from build123d import *

# Parameters (mm, degrees)
BOSS_EXTRUDE1_DEPTH      = 15
BOSS_EXTRUDE1_DEPTH_BACK = 15
SKETCH4_R                = 1.5
BOSS_EXTRUDE2_DEPTH      = 15
BOSS_EXTRUDE2_DEPTH_BACK = 15
SKETCH6_R                = 1.5


with BuildPart() as part:
    # Sketch1 → Revolve1 (revolve)
    with BuildSketch(Plane.XY, mode=Mode.PRIVATE) as revolve1_sk:
        with BuildLine():
            Line((-7.75, 54.212646434), (-7.75, 30.212646434))
            Line((-7.75, 30.212646434), (-3, 12.850690899))
            Line((-3, 12.850690899), (0, 12.850690899))
            Line((0, 12.850690899), (0, 67.181279304))
            ThreePointArc((0, 67.181279304), (-7.553938352, 62.895480825), (-7.75, 54.212646434))
        make_face()
    revolve(revolve1_sk.sketch.rotate(Axis((0, 0, 0), (0, 1, 0)), 270), axis=Axis((0, 0, 0), (0, 1, 0)))

    # Sketch4 → Boss-Extrude1 (add, two sides: drawn at the far end of the back side and taken through both)
    with BuildSketch(Plane.XY.offset(-BOSS_EXTRUDE1_DEPTH_BACK)):
        with Locations((0, 58.381279304)):
            Circle(SKETCH4_R)
    extrude(amount=BOSS_EXTRUDE1_DEPTH + BOSS_EXTRUDE1_DEPTH_BACK)

    # Sketch6 → Boss-Extrude2 (add, two sides: drawn at the far end of the back side and taken through both)
    with BuildSketch(Plane(origin=(0, 0, 0), x_dir=(0, 0, -1), z_dir=(1, 0, 0)).offset(-BOSS_EXTRUDE2_DEPTH_BACK)):
        with Locations((0, 58.381279304)):
            Circle(SKETCH6_R)
        with Locations((3, 47.381279304)):
            Circle(SKETCH6_R)
        with Locations((-3, 47.381279304)):
            Circle(SKETCH6_R)
    extrude(amount=BOSS_EXTRUDE2_DEPTH + BOSS_EXTRUDE2_DEPTH_BACK)


solid = part.part
Input: part model. Units: mm. Frame: model coordinates. A direction names the side the tool comes from. Give positions to 0.01 mm unless a question says otherwise; leave off trailing zeros. Loops run counter-clockwise (first coordinate to the right, second up) from the corner with the lowest first, then second, coordinate; pieces in that order, holes last. Notation, with made-up numbers: (16.25, 32) - (44.25, 32) arc R29 ccw to (44.25, 71) - close; hole circle Ø9 at (79, -16). An arc over 180 degrees is marked (long way). Use CSV: the item, a comma, the result in double quotes. Start each with the question number.
Item 1: Section B-B on x = 0. Return loops of the section in (y, z), then the cut area to 3 significant figures.
Item 2: Mould query, pull axis Z, two halves, no side actions, for faces 1 (the flat face through (-15, 58, 0)), 2 (the flat face through (0, 58, -15)), 3 (the cylindrical face through (11.79, 56.92, 0.33)), 4 (the cylindrical face through (10.6, 47.4, 4.5)). Classes: pulls with the +Z half, pulls with the -Z half, needs draft (parallel to the pull), parting line crosses it, or undercut.
Item 3: Contact query for flat-ended pins moving along their axis: P1, Ø12, axis at y = 29, z = -0.5, coming from the +X side; P2, Ø5, axis at x = 7.5, y = 54.5, coming from the +Z side; P3, Ø12, axis at x = -6, y = 43, coming from the -Z side. Output: stop coordinate, or through.
Item 4: Reachability of faces 5 (the cylindrical face through (10.594, 46.807, -4.386)), 6 (the cylindrical face through (-0.33, 56.92, 11.79)), 7 (the cylindrical face through (-0.33, 56.92, -11.88)), 8 (the flat face through (15, 47, 3)), 9 (the cylindrical face through (-11.88, 56.92, 0.33)) from +Z, -Z, +X, -X, +Y, -Y: full face, straight path, thin tool, end or side. Return the list, or none.
Item 5: Line query: line 1 (Z direction, x = 11.5, y = 47.5); line 2 (Z direction, x = -11.5, y = 48); line 3 (Z direction, x = 4.5, y = 42). Output: solid intervals per line, ascending.
Item 6: Section D-D on x = -10.5. Return loops of the section in (y, z).
Item 7: Section A-A on z = 0. Return loops of the section in (x, y).
Item 8: Section C-C on y = 37.5. Return loops of the section in (x, z), then the cut area to 3 significant figures.
Ans:
1,outline,"(12.85, -3) - (30.21, -7.75) - (54.21, -7.75) arc R8.8 ccw to (56.88, -8.67) - (56.88, -15) - (59.88, -15) - (59.88, -8.67) arc R8.8 ccw to (59.88, 8.67) - (59.88, 15) - (56.88, 15) - (56.88, 8.67) arc R8.8 ccw to (54.21, 7.75) - (30.21, 7.75) - (12.85, 3) - close"
1,area,"788 mm2"
2,face 1,"needs draft"
2,face 2,"pulls with the -Z half"
2,face 3,"parting line crosses it"
2,face 4,"undercut"
3,P1,"stops at x = 7.75"
3,P2,"stops at z = 6.49"
3,P3,"stops at z = -7.75"
4,face 5,"+X"
4,face 6,"+Z"
4,face 7,"-Z"
4,face 8,"+Z, -Z, +X, +Y, -Y"
4,face 9,"-X"
5,line 1,"z = -4.5 to -1.5, 1.5 to 4.5"
5,line 2,"z = -4.37 to -1.63, 1.63 to 4.37"
5,line 3,"z = -6.31 to 6.31"
6,outline,"circle Ø3 at (47.38, -3); circle Ø3 at (47.38, 3); circle Ø3 at (58.38, 0)"
7,outline,"(-15, 56.88) - (-8.67, 56.88) arc R8.8 ccw to (-7.75, 54.21) - (-7.75, 30.21) - (-3, 12.85) - (3, 12.85) - (7.75, 30.21) - (7.75, 54.21) arc R8.8 ccw to (8.67, 56.88) - (15, 56.88) - (15, 59.88) - (8.67, 59.88) arc R8.8 ccw to (-8.67, 59.88) - (-15, 59.88) - close"
8,outline,"circle Ø15.5 at (0, 0)"
8,area,"189 mm2"
